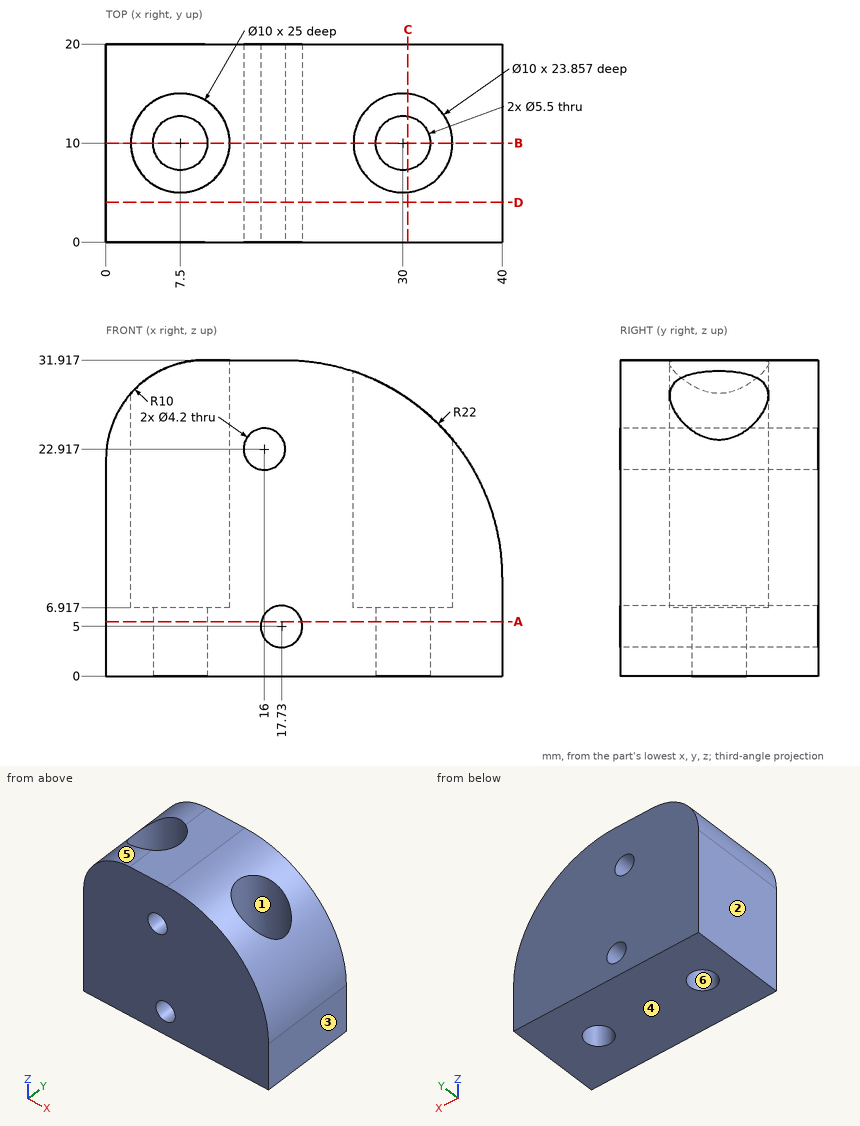
Print and shaded views of the part. All mm, measured from the part's lowest x, y and z. A direction names the side the tool comes from. Coordinates: 2 decimals unless noted, no trailing zeros. Order: outer loops, then holes, each group sorted by start corner. A loop starts at its lowest first (then second) coordinate and runs counter-clockwise, first axis right, second up.
Item 1: Saw through at C-C on x = 30.5. List the corners of the cut face in (y, z) (1 decimal).
Filled in:
outline: (0, 0) - (7.3, 0) - (7.3, 6.9) - (5, 6.9) - (5, 28) - (0, 28) - close; (12.7, 0) - (20, 0) - (20, 28) - (15, 28) - (15, 6.9) - (12.7, 6.9) - close
Item 2: Saw through at A-A on z = 5.5. List the corners of the cut face in (x, y), then the cut area to 3 significant figures.
Filled in:
outline: (0, 0) - (15.69, 0) - (15.69, 20) - (0, 20) - close; (19.77, 0) - (40, 0) - (40, 20) - (19.77, 20) - close; hole circle Ø5.5 at (7.5, 10); hole circle Ø5.5 at (30, 10)
area: 671 mm2
Item 3: Saw through at D-D on y = 4. List the corners of the cut face in (x, z), then the cut area to 3 significant figures.
Filled in:
outline: (0, 0) - (40, 0) - (40, 9.92) arc R22 ccw to (18, 31.92) - (10, 31.92) arc R10 ccw to (0, 21.92) - close; hole circle Ø4.2 at (16, 22.92); hole circle Ø4.2 at (17.73, 5)
area: 1,120 mm2
Item 4: Saw through at B-B on y = 10. List the corners of the cut face in (x, z).
Filled in:
outline: (0, 0) - (4.75, 0) - (4.75, 6.92) - (2.5, 6.92) - (2.5, 28.53) arc R10 ccw to (0, 21.92) - close; (10.25, 0) - (27.25, 0) - (27.25, 6.92) - (25, 6.92) - (25, 30.77) arc R22 ccw to (18, 31.92) - (12.5, 31.92) - (12.5, 6.92) - (10.25, 6.92) - close; (32.75, 0) - (40, 0) - (40, 9.92) arc R22 ccw to (35, 23.88) - (35, 6.92) - (32.75, 6.92) - close; hole circle Ø4.2 at (16, 22.92); hole circle Ø4.2 at (17.73, 5)
Item 5: Drop flat-ended pins along their axis: pin 1 Ø8 at (x, y) = (29, 12) entering from +Z; pin 2 Ø5 at (x, y) = (8.5, 8.5) entering from +Z; pin 3 Ø1.5 at (y, z) = (13, 16.5) entering from +X. Give the stop position or say it passes through.
Filled in:
pin 1: stops at z = 30.77
pin 2: stops at z = 6.92
pin 3: stops at x = 39.21
Item 6: Drill centre lines: L1, parallel to Z at x = 17.73, y = 11.5 (1 decimal); L2, parallel to Y at x = 7.5, z = 4.75; L3, parallel to X at y = 12, z = 24. Where is each one in solid material? Low to high.
Filled in:
L1: z = 0 to 2.9, 7.1 to 21.7, 24.1 to 31.9
L2: y = 0 to 7.25, 12.75 to 20
L3: x = 0.22 to 2.92, 12.08 to 14.2, 17.8 to 25.42, 34.58 to 34.9
Item 7: Tool access for the marked faces 1 and 2: list every direction of +Z, -Z, +X, -X, +Y, -Y with a clear straight run to the whole face (end or side of a thin tool).
Filled in:
face 1: +Z
face 2: +Z, -Z, -X, +Y, -Y
Item 8: Mould opens along X. For the marked faces 3, 4, 5 and 6 say: released by +X, released by -X, zero draft, split by the parting line, or undercut.
Filled in:
face 3: released by +X
face 4: zero draft
face 5: released by -X
face 6: undercut
